from build123d import *

# Parameters (mm, degrees)
BOSS_EXTRU_1_DEPTH = 3.5
BOSS_EXTRU_2_DEPTH = 6


with BuildPart() as part:
    # Esquisse1 → Boss.-Extru.1 (new body)
    with BuildSketch(Plane.XY):
        Polygon((-45.75, 14.450660172), (-14.450660172, 45.75), (14.450660172, 45.75), (45.75, 14.450660172), (45.75, -14.450660172), (14.450660172, -45.75), (-14.450660172, -45.75), (-45.75, -14.450660172), align=None)
        with BuildLine():
            Line((-13.017835842, 13.017835842), (-2.057680733, 23.97799095))
            ThreePointArc((-2.057680733, 23.97799095), (-1.325447686, 25.745757903), (-2.057680733, 27.513524856))
            Line((-2.057680733, 27.513524856), (-7.360981592, 32.816825715))
            ThreePointArc((-7.360981592, 32.816825715), (-9.128748545, 33.549058762), (-10.896515498, 32.816825715))
            Line((-10.896515498, 32.816825715), (-32.816825715, 10.896515498))
            ThreePointArc((-32.816825715, 10.896515498), (-33.549058762, 9.128748545), (-32.816825715, 7.360981592))
            Line((-32.816825715, 7.360981592), (-27.513524856, 2.057680733))
            ThreePointArc((-27.513524856, 2.057680733), (-25.745757903, 1.325447686), (-23.97799095, 2.057680733))
            Line((-23.97799095, 2.057680733), (-13.017835842, 13.017835842))
        make_face(mode=Mode.SUBTRACT)
        with BuildLine():
            Line((-13.017835842, -13.017835842), (-21.856670606, -4.179001077))
            ThreePointArc((-21.856670606, -4.179001077), (-23.624437559, -3.44676803), (-25.392204512, -4.179001077))
            Line((-25.392204512, -4.179001077), (-30.695505371, -9.482301936))
            ThreePointArc((-30.695505371, -9.482301936), (-31.427738418, -11.250068889), (-30.695505371, -13.017835842))
            Line((-30.695505371, -13.017835842), (-13.017835842, -30.695505371))
            ThreePointArc((-13.017835842, -30.695505371), (-11.250068889, -31.427738418), (-9.482301936, -30.695505371))
            Line((-9.482301936, -30.695505371), (-4.179001077, -25.392204512))
            ThreePointArc((-4.179001077, -25.392204512), (-3.44676803, -23.624437559), (-4.179001077, -21.856670606))
            Line((-4.179001077, -21.856670606), (-13.017835842, -13.017835842))
        make_face(mode=Mode.SUBTRACT)
        with BuildLine():
            Line((27.513524856, -2.057680733), (32.816825715, -7.360981592))
            ThreePointArc((32.816825715, -7.360981592), (33.549058762, -9.128748545), (32.816825715, -10.896515498))
            Line((32.816825715, -10.896515498), (10.896515498, -32.816825715))
            ThreePointArc((10.896515498, -32.816825715), (9.128748545, -33.549058762), (7.360981592, -32.816825715))
            Line((7.360981592, -32.816825715), (2.057680733, -27.513524856))
            ThreePointArc((2.057680733, -27.513524856), (1.325447686, -25.745757903), (2.057680733, -23.97799095))
            Line((2.057680733, -23.97799095), (13.017835842, -13.017835842))
            Line((13.017835842, -13.017835842), (23.97799095, -2.057680733))
            ThreePointArc((23.97799095, -2.057680733), (25.745757903, -1.325447686), (27.513524856, -2.057680733))
        make_face(mode=Mode.SUBTRACT)
        with BuildLine():
            Line((4.179001077, 25.392204512), (9.482301936, 30.695505371))
            ThreePointArc((9.482301936, 30.695505371), (11.250068889, 31.427738418), (13.017835842, 30.695505371))
            Line((13.017835842, 30.695505371), (30.695505371, 13.017835842))
            ThreePointArc((30.695505371, 13.017835842), (31.427738418, 11.250068889), (30.695505371, 9.482301936))
            Line((30.695505371, 9.482301936), (25.392204512, 4.179001077))
            ThreePointArc((25.392204512, 4.179001077), (23.624437559, 3.44676803), (21.856670606, 4.179001077))
            Line((21.856670606, 4.179001077), (13.017835842, 13.017835842))
            Line((13.017835842, 13.017835842), (4.179001077, 21.856670606))
            ThreePointArc((4.179001077, 21.856670606), (3.44676803, 23.624437559), (4.179001077, 25.392204512))
        make_face(mode=Mode.SUBTRACT)
    extrude(amount=BOSS_EXTRU_1_DEPTH)

    # Esquisse2 → Boss.-Extru.2 (add)
    with BuildSketch(Plane.XY):
        Polygon((-48.75, -15.693300859), (-48.75, 15.693300859), (-15.693300859, 48.75), (15.693300859, 48.75), (48.75, 15.693300859), (48.75, -15.693300859), (15.693300859, -48.75), (-15.693300859, -48.75), align=None)
        Polygon((-45.75, 14.450660172), (-14.450660172, 45.75), (14.450660172, 45.75), (45.75, 14.450660172), (45.75, -14.450660172), (14.450660172, -45.75), (-14.450660172, -45.75), (-45.75, -14.450660172), align=None, mode=Mode.SUBTRACT)
    extrude(amount=BOSS_EXTRU_2_DEPTH)


solid = part.part
Can you work these out from the model? Positions are in its coordinate system, mm. A direction names the side the tool comes from. Coordinates: 2 decimals unless noted, no trailing zeros. Loops run counter-clockwise (first coordinate to the right, second up) from the corner with the lowest first, then second, coordinate; pieces in that order, holes last. Notation, with made-up numbers: (35, 34.25) - (43, 34.25) arc R9 ccw to (43, 47.25) - close; hole circle Ø3 at (39.5, -31.75). An arc over 180 degrees is marked (long way). Answer as a JSON object with one key per item and string values. Group by question number.
Item 1: If we section it at D-D (z = 2.2): State how many separate pieces and enclosed holes the cut face has, plus the area to 3 significant figures.
Item 2: If we section it at A-A (x = -18): List the corners of the cut face in (y, z) for me.
Item 3: If we section it at C-C (x = 39): List the corners of the cut face in (y, z) for me, plus the area to 3 significant figures.
Item 4: On a 3-axis mill with a long thin cutter (end or side, diameter ignored), from which of +Z, -Z, +X, -X, +Y, -Y can I reach the whole of each face in a straight line? I mean faces 5 (the face through (9.16, -33.55, 1.73)), 6 (the face through (-31.99, -32.453, 2.958)), 7 (the face through (0, -45.75, 5)). Say none if no direction works.
Item 5: If I drill on L1, parallel to Y at x = 18.5, z = 1.5; L2, parallel to Y at x = -6, z = 1.65; L3, parallel to X at y = -10, z = 0.5, over which ranges is the centre line in solid material (lowest first)? Write a range as from..to.
Item 6: For pin 1 (1 mm diameter, centred on x = 36, z = 4, fed in from +Y), with a flat end and sliding along its axis, tell me the tip position at first contact or that it passes through.
Item 7: If we mould it in two halves opening along X, with no side actions, what happens to faces 1 (the face through (-48.75, 0, 3)), 2 (the face through (1, 1, 0)), 3 (the face through (4.746, -30.202, 1.726)), 4 (the face through (-30.202, 4.746, 1.726))? For each: released by +X, released by -X, zero draft, split by the parting line, or undercut.
Returned:
{
 "1": {"separate pieces": "1", "enclosed holes": "4", "area": "5,690 mm²"},
 "2": {"outline": "(-46.44, 0) - (-25.71, 0) - (-25.71, 3.5) - (-42.2, 3.5) - (-42.2, 6) - (-46.44, 6) - close; (-8.04, 0) - (8.04, 0) - (8.04, 3.5) - (-8.04, 3.5) - close; (25.71, 0) - (46.44, 0) - (46.44, 6) - (42.2, 6) - (42.2, 3.5) - (25.71, 3.5) - close"},
 "3": {"outline": "(-25.44, 0) - (25.44, 0) - (25.44, 6) - (21.2, 6) - (21.2, 3.5) - (-21.2, 3.5) - (-21.2, 6) - (-25.44, 6) - close", "area": "199 mm²"},
 "4": {"face 5": "+Z, -Z", "face 6": "+Z, -Z, -X, -Y", "face 7": "+Z"},
 "5": {"L1": "y = -45.94..-25.21, -7.54..7.54, 25.21..45.94", "L2": "y = -48.75..-27.21, -20.04..20.04, 31.46..48.75", "L3": "x = -48.75..-31.09, -16.04..16.04, 33.39..48.75"},
 "6": {"pin 1": "stops at y = 28.94"},
 "7": {"face 1": "released by -X", "face 2": "zero draft", "face 3": "undercut", "face 4": "undercut"}
}
